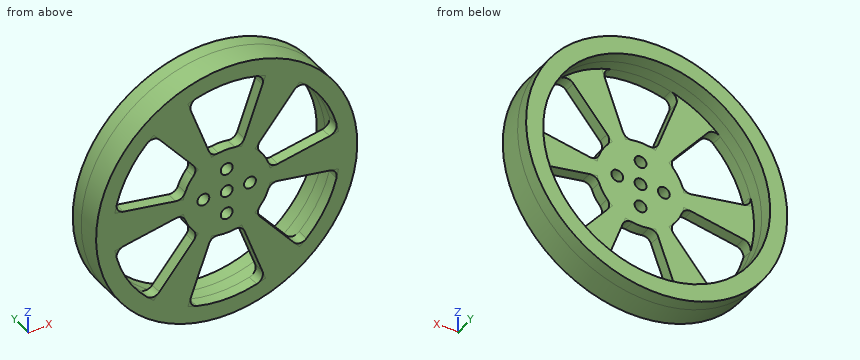
from build123d import *
from build123d.topology import SkipClean

# Parameters (mm, degrees)
SKETCH1_R            = 24.257
BOSS_EXTRUDE1_DEPTH  = 4.445
M2_CLEARANCE_HOLE1_D = 2.2
SKETCH4_R            = 21.082
CUT_EXTRUDE1_DEPTH   = 2.286
CUT_EXTRUDE2_DEPTH   = 35.380661628
FILLET1_DEPTH        = 2.159
BOSS_EXTRUDE2_START  = 2.54
SKETCH6_R            = 24.257
SKETCH6_R_2          = 21.082
BOSS_EXTRUDE2_DEPTH  = 2.54


with BuildPart() as part:
    # Sketch1 → Boss-Extrude1 (new body)
    with BuildSketch(Plane(origin=(0, 0, 0), x_dir=(1, 0, 0), z_dir=(0, 1, 0))):
        with Locations(Location((0, 0, 0), (0, 0, 270))):
            Circle(SKETCH1_R)
    extrude(amount=BOSS_EXTRUDE1_DEPTH)

    # M2 Clearance Hole1 (through all)
    with Locations(Plane(origin=(0, 4.445, 0), x_dir=(1, 0, 0), z_dir=(0, 1, 0))):
        with Locations((0, 0), (0, 4.32848345), (0, -4.32848345), (-4.32848345, 0), (4.32848345, 0)):
            Hole(M2_CLEARANCE_HOLE1_D / 2)

    # Sketch4 → Cut-Extrude1 (cut)
    with BuildSketch(Plane(origin=(0, 4.445, 0), x_dir=(1, 0, 0), z_dir=(0, 1, 0))):
        with Locations(Location((0, 0, 0), (0, 0, 270))):
            Circle(SKETCH4_R)
    extrude(amount=-CUT_EXTRUDE1_DEPTH, mode=Mode.SUBTRACT)

    # Sketch5 → Cut-Extrude2 (cut, through all)
    with SkipClean():  # the faces are left unmerged after this step: merging them gives an invalid solid
        with BuildSketch(Plane(origin=(0, 2.159, 0), x_dir=(1, 0, 0), z_dir=(0, 1, 0))):
            with BuildLine():
                Line((-2.790798865, 7.667656862), (-7.210468662, 19.810599831))
                ThreePointArc((-7.210468662, 19.810599831), (0, 21.082), (7.210468662, 19.810599831))
                Line((7.210468662, 19.810599831), (2.790798865, 7.667656862))
                ThreePointArc((2.790798865, 7.667656862), (0, 8.15975), (-2.790798865, 7.667656862))
            make_face()
            with BuildLine():
                Line((5.244986198, 6.250731145), (13.551248387, 16.14974895))
                ThreePointArc((13.551248387, 16.14974895), (18.257547563, 10.541), (20.761717049, 3.660850882))
                Line((20.761717049, 3.660850882), (8.035785063, 1.416925718))
                ThreePointArc((8.035785063, 1.416925718), (7.066550789, 4.079875), (5.244986198, 6.250731145))
            make_face()
            with BuildLine():
                Line((8.035785063, -1.416925718), (20.761717049, -3.660850882))
                ThreePointArc((20.761717049, -3.660850882), (18.257547563, -10.541), (13.551248387, -16.14974895))
                Line((13.551248387, -16.14974895), (5.244986198, -6.250731145))
                ThreePointArc((5.244986198, -6.250731145), (7.066550789, -4.079875), (8.035785063, -1.416925718))
            make_face()
            with BuildLine():
                Line((2.790798865, -7.667656862), (7.210468662, -19.810599831))
                ThreePointArc((7.210468662, -19.810599831), (0, -21.082), (-7.210468662, -19.810599831))
                Line((-7.210468662, -19.810599831), (-2.790798865, -7.667656862))
                ThreePointArc((-2.790798865, -7.667656862), (0, -8.15975), (2.790798865, -7.667656862))
            make_face()
            with BuildLine():
                Line((-5.244986198, -6.250731145), (-13.551248387, -16.14974895))
                ThreePointArc((-13.551248387, -16.14974895), (-18.257547563, -10.541), (-20.761717049, -3.660850882))
                Line((-20.761717049, -3.660850882), (-8.035785063, -1.416925718))
                ThreePointArc((-8.035785063, -1.416925718), (-7.066550789, -4.079875), (-5.244986198, -6.250731145))
            make_face()
            with BuildLine():
                Line((-8.035785063, 1.416925718), (-20.761717049, 3.660850882))
                ThreePointArc((-20.761717049, 3.660850882), (-18.257547563, 10.541), (-13.551248387, 16.14974895))
                Line((-13.551248387, 16.14974895), (-5.244986198, 6.250731145))
                ThreePointArc((-5.244986198, 6.250731145), (-7.066550789, 4.079875), (-8.035785063, 1.416925718))
            make_face()
        extrude(amount=-CUT_EXTRUDE2_DEPTH, mode=Mode.SUBTRACT)

    # Fillet1: read off the stored shape, not the designer's step
    # Fillet1 outline → Fillet1 (add)
    with SkipClean():  # the faces are left unmerged after this step: merging them gives an invalid solid
        with BuildSketch(Plane(origin=(0, 0, 0), x_dir=(1, 0, 0), z_dir=(0, 1, 0))):
            with BuildLine():
                ThreePointArc((-5.573280223, -20.331976578), (-6.563834268, -19.529933732), (-6.645367543, -18.257997268))
                Line((-6.645367543, -18.257997268), (-7.210468662, -19.810599831))
                ThreePointArc((-7.210468662, -19.810599831), (-6.397188235, -20.087974181), (-5.573280223, -20.331976578))
            make_face()
            with BuildLine():
                Line((-2.790798865, -7.667656862), (-3.289243946, -9.037123468))
                ThreePointArc((-3.289243946, -9.037123468), (-2.583701402, -8.200944789), (-1.504732413, -8.019806757))
                ThreePointArc((-1.504732413, -8.019806757), (-2.154970911, -7.870045771), (-2.790798865, -7.667656862))
            make_face()
            with BuildLine():
                ThreePointArc((6.645367543, -18.257997268), (6.563834268, -19.529933732), (5.573280223, -20.331976578))
                ThreePointArc((5.573280223, -20.331976578), (6.397188235, -20.087974181), (7.210468662, -19.810599831))
                Line((7.210468662, -19.810599831), (6.645367543, -18.257997268))
            make_face()
            with BuildLine():
                ThreePointArc((-14.821368114, -14.992590544), (-14.198101834, -15.584114615), (-13.551248387, -16.14974895))
                Line((-13.551248387, -16.14974895), (-12.489205685, -14.884055743))
                ThreePointArc((-12.489205685, -14.884055743), (-13.631501612, -15.449414088), (-14.821368114, -14.992590544))
            make_face()
            with BuildLine():
                ThreePointArc((2.790798865, -7.667656862), (2.154970911, -7.870045771), (1.504732413, -8.019806757))
                ThreePointArc((1.504732413, -8.019806757), (2.583701402, -8.200944789), (3.289243946, -9.037123468))
                Line((3.289243946, -9.037123468), (2.790798865, -7.667656862))
            make_face()
            with BuildLine():
                Line((12.489205685, -14.884055743), (13.551248387, -16.14974895))
                ThreePointArc((13.551248387, -16.14974895), (14.198101834, -15.584114615), (14.821368114, -14.992590544))
                ThreePointArc((14.821368114, -14.992590544), (13.631501612, -15.449414088), (12.489205685, -14.884055743))
            make_face()
            with BuildLine():
                ThreePointArc((-6.192990179, -5.313039875), (-5.810375821, -6.338023444), (-6.181756528, -7.36713055))
                Line((-6.181756528, -7.36713055), (-5.244986198, -6.250731145))
                ThreePointArc((-5.244986198, -6.250731145), (-5.738174111, -5.801282439), (-6.192990179, -5.313039875))
            make_face()
            with BuildLine():
                ThreePointArc((-20.761717049, -3.660850882), (-20.595290068, -4.503859567), (-20.394648337, -5.339386034))
                ThreePointArc((-20.394648337, -5.339386034), (-20.19533588, -4.080519643), (-19.134573227, -3.373941524))
                Line((-19.134573227, -3.373941524), (-20.761717049, -3.660850882))
            make_face()
            with BuildLine():
                Line((5.244986198, -6.250731145), (6.181756528, -7.36713055))
                ThreePointArc((6.181756528, -7.36713055), (5.810375821, -6.338023444), (6.192990179, -5.313039875))
                ThreePointArc((6.192990179, -5.313039875), (5.738174111, -5.801282439), (5.244986198, -6.250731145))
            make_face()
            with BuildLine():
                ThreePointArc((19.134573227, -3.373941524), (20.19533588, -4.080519643), (20.394648337, -5.339386034))
                ThreePointArc((20.394648337, -5.339386034), (20.595290068, -4.503859567), (20.761717049, -3.660850882))
                Line((20.761717049, -3.660850882), (19.134573227, -3.373941524))
            make_face()
            with BuildLine():
                ThreePointArc((-9.471000473, -1.669992918), (-8.394077223, -1.862921344), (-7.697722592, -2.706766883))
                ThreePointArc((-7.697722592, -2.706766883), (-7.893145022, -2.068763332), (-8.035785063, -1.416925718))
                Line((-8.035785063, -1.416925718), (-9.471000473, -1.669992918))
            make_face()
            with BuildLine():
                ThreePointArc((-20.394648337, 5.339386034), (-20.595290068, 4.503859567), (-20.761717049, 3.660850882))
                Line((-20.761717049, 3.660850882), (-19.134573227, 3.373941524))
                ThreePointArc((-19.134573227, 3.373941524), (-20.19533588, 4.080519643), (-20.394648337, 5.339386034))
            make_face()
            with BuildLine():
                ThreePointArc((8.035785063, -1.416925718), (7.893145022, -2.068763332), (7.697722592, -2.706766883))
                ThreePointArc((7.697722592, -2.706766883), (8.394077223, -1.862921344), (9.471000473, -1.669992918))
                Line((9.471000473, -1.669992918), (8.035785063, -1.416925718))
            make_face()
            with BuildLine():
                ThreePointArc((-7.697722592, 2.706766883), (-8.394077223, 1.862921344), (-9.471000473, 1.669992918))
                Line((-9.471000473, 1.669992918), (-8.035785063, 1.416925718))
                ThreePointArc((-8.035785063, 1.416925718), (-7.893145022, 2.068763332), (-7.697722592, 2.706766883))
            make_face()
            with BuildLine():
                ThreePointArc((-13.551248387, 16.14974895), (-14.198101834, 15.584114615), (-14.821368114, 14.992590544))
                ThreePointArc((-14.821368114, 14.992590544), (-13.631501612, 15.449414088), (-12.489205685, 14.884055743))
                Line((-12.489205685, 14.884055743), (-13.551248387, 16.14974895))
            make_face()
            with BuildLine():
                Line((19.134573227, 3.373941524), (20.761717049, 3.660850882))
                ThreePointArc((20.761717049, 3.660850882), (20.595290068, 4.503859567), (20.394648337, 5.339386034))
                ThreePointArc((20.394648337, 5.339386034), (20.19533588, 4.080519643), (19.134573227, 3.373941524))
            make_face()
            with BuildLine():
                ThreePointArc((-6.181756528, 7.36713055), (-5.810375821, 6.338023444), (-6.192990179, 5.313039875))
                ThreePointArc((-6.192990179, 5.313039875), (-5.738174111, 5.801282439), (-5.244986198, 6.250731145))
                Line((-5.244986198, 6.250731145), (-6.181756528, 7.36713055))
            make_face()
            with BuildLine():
                ThreePointArc((-5.573280223, 20.331976578), (-6.397188235, 20.087974181), (-7.210468662, 19.810599831))
                Line((-7.210468662, 19.810599831), (-6.645367543, 18.257997268))
                ThreePointArc((-6.645367543, 18.257997268), (-6.563834268, 19.529933732), (-5.573280223, 20.331976578))
            make_face()
            with BuildLine():
                Line((8.035785063, 1.416925718), (9.471000473, 1.669992918))
                ThreePointArc((9.471000473, 1.669992918), (8.394077223, 1.862921344), (7.697722592, 2.706766883))
                ThreePointArc((7.697722592, 2.706766883), (7.893145022, 2.068763332), (8.035785063, 1.416925718))
            make_face()
            with BuildLine():
                ThreePointArc((12.489205685, 14.884055743), (13.631501612, 15.449414088), (14.821368114, 14.992590544))
                ThreePointArc((14.821368114, 14.992590544), (14.198101834, 15.584114615), (13.551248387, 16.14974895))
                Line((13.551248387, 16.14974895), (12.489205685, 14.884055743))
            make_face()
            with BuildLine():
                ThreePointArc((-1.504732413, 8.019806757), (-2.583701402, 8.200944789), (-3.289243946, 9.037123468))
                Line((-3.289243946, 9.037123468), (-2.790798865, 7.667656862))
                ThreePointArc((-2.790798865, 7.667656862), (-2.154970911, 7.870045771), (-1.504732413, 8.019806757))
            make_face()
            with BuildLine():
                ThreePointArc((7.210468662, 19.810599831), (6.397188235, 20.087974181), (5.573280223, 20.331976578))
                ThreePointArc((5.573280223, 20.331976578), (6.563834268, 19.529933732), (6.645367543, 18.257997268))
                Line((6.645367543, 18.257997268), (7.210468662, 19.810599831))
            make_face()
            with BuildLine():
                ThreePointArc((5.244986198, 6.250731145), (5.738174111, 5.801282439), (6.192990179, 5.313039875))
                ThreePointArc((6.192990179, 5.313039875), (5.810375821, 6.338023444), (6.181756528, 7.36713055))
                Line((6.181756528, 7.36713055), (5.244986198, 6.250731145))
            make_face()
            with BuildLine():
                ThreePointArc((3.289243946, 9.037123468), (2.583701402, 8.200944789), (1.504732413, 8.019806757))
                ThreePointArc((1.504732413, 8.019806757), (2.154970911, 7.870045771), (2.790798865, 7.667656862))
                Line((2.790798865, 7.667656862), (3.289243946, 9.037123468))
            make_face()
        extrude(amount=FILLET1_DEPTH)

    # Sketch6 → Boss-Extrude2 (add)
    with SkipClean():  # the faces are left unmerged after this step: merging them gives an invalid solid
        with BuildSketch(Plane(origin=(0, 4.445, 0), x_dir=(1, 0, 0), z_dir=(0, 1, 0)).offset(BOSS_EXTRUDE2_START)):
            with Locations(Location((0, 0, 0), (0, 0, 270))):
                Circle(SKETCH6_R)
            with Locations(Location((0, 0, 0), (0, 0, 270))):
                Circle(SKETCH6_R_2, mode=Mode.SUBTRACT)
        extrude(amount=-BOSS_EXTRUDE2_DEPTH)


solid = part.part
Source: CAD feature listing. Evaluate the final solid. Frame: model axes, mm. Give positions to 0.01 mm unless a question says otherwise; leave off trailing zeros. Order: outer loops, then holes, each group sorted by start corner. A loop starts at its lowest first (then second) coordinate and runs counter-clockwise, first axis right, second up. Notation, with made-up numbers: (72.5, 42) -> (110.5, 42) arc R24 cw to (110.5, 62) -> close; hole circle Ø4 at (-23.5, 84.25). An arc over 180 degrees is marked (long way). Use a Markdown table: item, result.
1) Section query A-A, the plane z = 0. Return the cut outline in (x, y) (3 decimals).
Answer list:
| item | result |
|---|---|
| outline | (-24.257, 0) -> (-5.428, 0) -> (-5.428, 2.159) -> (-21.082, 2.159) -> (-21.082, 6.985) -> (-24.257, 6.985) -> close; (-3.228, 0) -> (-1.1, 0) -> (-1.1, 2.159) -> (-3.228, 2.159) -> close; (1.1, 0) -> (3.228, 0) -> (3.228, 2.159) -> (1.1, 2.159) -> close; (5.428, 0) -> (24.257, 0) -> (24.257, 6.985) -> (21.082, 6.985) -> (21.082, 2.159) -> (5.428, 2.159) -> close |
2) Contact query for flat-ended pins moving along their axis: P1, Ø0.8, axis at x = -6.5, z = 19.5, coming from the +Y side; P2, Ø4, axis at x = -8.5, y = 3, coming from the -Z side; P3, Ø3, axis at x = 7.5, y = 6, coming from the +Z side. Output: stop coordinate, or through.
Answer list:
| item | result |
|---|---|
| P1 | y = 2.16 |
| P2 | z = -23.37 |
| P3 | z = 23.5 |
3) Section query D-D, the plane y = 3.25. Return the cut outline in (x, z).
Answer list:
| item | result |
|---|---|
| outline | circle Ø48.51 at (0, 0); hole circle Ø42.16 at (0, 0) |
4) Ray query, line 1 along X through (y, z) = (4, 0); line 2 along X through (y, z) = (0.5, 12); line 3 along Z through (x, y) = (-14.5, 2). Return the intervals inside material, ascending. Write a range as [from, to].
Answer list:
| item | result |
|---|---|
| line 1 | [-24.26, -21.08], [21.08, 24.26] |
| line 2 | [-21.08, -17.33], [-10.07, -4.37], [4.37, 10.07], [17.33, 21.08] |
| line 3 | [-19.45, -15.24], [-2.56, 2.56], [15.24, 19.45] |
5) Section query C-C, the plane x = 0. Return the cut outline in (y, z) (3 decimals), then the cut area to 3 significant figures.
Answer list:
| item | result |
|---|---|
| outline | (0, -24.257) -> (6.985, -24.257) -> (6.985, -21.082) -> (0, -21.082) -> close; (0, -8.16) -> (2.159, -8.16) -> (2.159, -5.428) -> (0, -5.428) -> close; (0, -3.228) -> (2.159, -3.228) -> (2.159, -1.1) -> (0, -1.1) -> close; (0, 1.1) -> (2.159, 1.1) -> (2.159, 3.228) -> (0, 3.228) -> close; (0, 5.428) -> (2.159, 5.428) -> (2.159, 8.16) -> (0, 8.16) -> close; (0, 21.082) -> (6.985, 21.082) -> (6.985, 24.257) -> (0, 24.257) -> close |
| area | 65.3 mm² |
6) Section query B-B, the plane x = 16. Return the cut outline in (y, z) (3 decimals), then the cut area to 3 significant figures.
Answer list:
| item | result |
|---|---|
| outline | (0, -18.232) -> (6.985, -18.232) -> (6.985, -13.728) -> (0, -13.728) -> close; (0, -2.821) -> (2.159, -2.821) -> (2.159, 2.821) -> (0, 2.821) -> close; (0, 13.728) -> (6.985, 13.728) -> (6.985, 18.232) -> (0, 18.232) -> close |
| area | 75.1 mm² |
